Autodesk Inventor part; units mm, degrees
ref_plane "YZ Plane" through (0, 0, 0) normal (1, 0, 0) x (0, 1, 0)
ref_plane "XZ Plane" through (0, 0, 0) normal (0, 1, 0) x (-1, 0, 0)
ref_plane "XY Plane" through (0, 0, 0) normal (0, 0, 1) x (1, 0, 0)
sketch "Sketch3" plane through (0, 0, 0) normal (0, 1, 0) x (-1, 0, 0)
  line L0 (72.5, 90) -> (-72.5, 90)
  line L1 (-72.5, 90) -> (-72.5, -90)
  line L2 (-72.5, -90) -> (72.5, -90)
  line L3 (72.5, -90) -> (72.5, 90)
  line L4 (72.5, 90) -> (-72.5, -90) construction
  line L5 (-72.5, 90) -> (72.5, -90) construction
  point P0 (0, 0)
  dimension "d7" = 145
  dimension "d8" = 180
extrude "Extrusion3" add sketch "Sketch3" along normal blind 5
sketch "Sketch4" plane through (0, 5, 0) normal (0, 1, 0) x (1, 0, 0)
  line L0 (23.935, -64) -> (72.5, -64)
  line L1 (72.5, -64) -> (72.5, -26.408)
  line L2 (72.5, -26.408) -> (23.935, -26.408)
  line L3 (23.935, -26.408) -> (23.935, -64)
  line L4 (23.935, -64) -> (72.5, -26.408) construction
  line L5 (72.5, -64) -> (23.935, -26.408) construction
  line L6 (72.5, -90) -> (72.5, 90)
  line L7 (-72.5, -90) -> (72.5, -90)
  line L8 (-72.5, -64) -> (-23.935, -64)
  line L9 (-23.935, -64) -> (-23.935, -26.408)
  line L10 (-23.935, -26.408) -> (-72.5, -26.408)
  line L11 (-72.5, -26.408) -> (-72.5, -64)
  line L12 (-72.5, -64) -> (-23.935, -26.408) construction
  line L13 (-23.935, -64) -> (-72.5, -26.408) construction
  line L14 (-72.5, 90) -> (-72.5, -90)
  point P0 (0, 0)
  point P1 (48.2175, -45.204)
  point P2 (-48.2175, -45.204)
  dimension "d11" = 48.565
  dimension "d12" = 37.592
  dimension "d13" = 0
  dimension "d14" = 26
  dimension "d20" = 48.565
  dimension "d21" = 37.592
  dimension "d22" = 0
  dimension "d23" = 26
extrude "Extrusion4" cut sketch "Sketch4" against normal blind 2
sketch "Sketch5" plane through (0, 3, 0) normal (0, 1, 0) x (1, 0, 0)
  circle A0 centre (66.797, -60.825) radius 1.588
  line L0 (72.5, -26.408) -> (72.5, -64)
  line L1 (72.5, -64) -> (23.935, -64)
  circle A1 centre (60.447, -60.825) radius 1.588
  circle A2 centre (54.097, -60.825) radius 1.588
  circle A3 centre (47.747, -60.825) radius 1.588
  circle A4 centre (41.397, -60.825) radius 1.588
  circle A5 centre (35.047, -60.825) radius 1.588
  circle A6 centre (28.697, -60.825) radius 1.588
  circle A7 centre (66.797, -29.583) radius 1.588
  circle A8 centre (60.447, -29.583) radius 1.588
  circle A9 centre (54.097, -29.583) radius 1.588
  circle A10 centre (47.747, -29.583) radius 1.588
  circle A11 centre (41.397, -29.583) radius 1.588
  circle A12 centre (35.047, -29.583) radius 1.588
  circle A13 centre (28.697, -29.583) radius 1.588
  circle A14 centre (-66.797, -60.825) radius 1.588
  line L2 (-23.935, -64) -> (-72.5, -64)
  line L3 (-72.5, -64) -> (-72.5, -26.408)
  circle A15 centre (-60.447, -60.825) radius 1.588
  circle A16 centre (-54.097, -60.825) radius 1.588
  circle A17 centre (-47.747, -60.825) radius 1.588
  circle A18 centre (-41.397, -60.825) radius 1.588
  circle A19 centre (-35.047, -60.825) radius 1.588
  circle A20 centre (-28.697, -60.825) radius 1.588
  circle A21 centre (-66.797, -29.583) radius 1.588
  circle A22 centre (-60.447, -29.583) radius 1.588
  circle A23 centre (-54.097, -29.583) radius 1.588
  circle A24 centre (-47.747, -29.583) radius 1.588
  circle A25 centre (-41.397, -29.583) radius 1.588
  circle A26 centre (-35.047, -29.583) radius 1.588
  circle A27 centre (-28.697, -29.583) radius 1.588
  point P0 (0, 0)
  dimension "d24" = 3.176
  dimension "d25" = 5.703
  dimension "d26" = 3.175
  dimension "d30" = 6.35
  dimension "d33" = 31.242
  dimension "d36" = 3.176
  dimension "d37" = 3.175
  dimension "d38" = 5.703
  dimension "d41" = 6.35
  dimension "d44" = 31.242
extrude "Extrusion5" cut sketch "Sketch5" against normal through all
sketch "Sketch6" plane through (0, 5, 0) normal (0, 1, 0) x (1, 0, 0)
  line L0 (42.5, 32.6926) -> (52.5, 32.6926)
  line L1 (52.5, 32.6926) -> (52.5, 37.6926)
  line L2 (52.5, 37.6926) -> (42.5, 37.6926)
  line L3 (42.5, 37.6926) -> (42.5, 32.6926)
  line L4 (42.5, 32.6926) -> (52.5, 37.6926) construction
  line L5 (52.5, 32.6926) -> (42.5, 37.6926) construction
  line L6 (72.5, -26.408) -> (72.5, 90)
  line L7 (-52.5, 32.6926) -> (-42.5, 32.6926)
  line L8 (-42.5, 32.6926) -> (-42.5, 37.6926)
  line L9 (-42.5, 37.6926) -> (-52.5, 37.6926)
  line L10 (-52.5, 37.6926) -> (-52.5, 32.6926)
  line L11 (-52.5, 32.6926) -> (-42.5, 37.6926) construction
  line L12 (-42.5, 32.6926) -> (-52.5, 37.6926) construction
  line L13 (-72.5, 90) -> (-72.5, -26.408)
  line L14 (-52.5, -15.3074) -> (-42.5, -15.3074)
  line L15 (-42.5, -15.3074) -> (-42.5, -12.3074)
  line L16 (-42.5, -12.3074) -> (-52.5, -12.3074)
  line L17 (-52.5, -12.3074) -> (-52.5, -15.3074)
  line L18 (-52.5, -15.3074) -> (-42.5, -12.3074) construction
  line L19 (-42.5, -15.3074) -> (-52.5, -12.3074) construction
  line L20 (42.5, -15.3074) -> (52.5, -15.3074)
  line L21 (52.5, -15.3074) -> (52.5, -12.3074)
  line L22 (52.5, -12.3074) -> (42.5, -12.3074)
  line L23 (42.5, -12.3074) -> (42.5, -15.3074)
  line L24 (42.5, -15.3074) -> (52.5, -12.3074) construction
  line L25 (52.5, -15.3074) -> (42.5, -12.3074) construction
  arc A0 (-42.5, 37.6926) -> (-52.5, 37.6926) centre (-47.5, 37.6926) ccw
  arc A1 (52.5, 37.6926) -> (42.5, 37.6926) centre (47.5, 37.6926) ccw
  line L26 (-72.5, -26.408) -> (-23.935, -26.408)
  line L27 (23.935, -26.408) -> (72.5, -26.408)
  point P0 (0, 0)
  point P1 (47.5, 35.1926)
  point P2 (-47.5, 35.1926)
  point P3 (-47.5, -13.8074)
  point P4 (47.5, -13.8074)
  dimension "d49" = 10
  dimension "d50" = 5
  dimension "d51" = 20
  dimension "d52" = 10
  dimension "d53" = 5
  dimension "d54" = 20
  dimension "d57" = 10
  dimension "d58" = 3
  dimension "d59" = 10
  dimension "d60" = 3
  dimension "d61" = 45
  dimension "d84" = 11.1006
  dimension "d85" = 11.1006
extrude "Extrusion6" add sketch "Sketch6" along normal blind 24
sketch "Sketch7" plane through (0, 5, 0) normal (0, 1, 0) x (1, 0, 0)
  circle A0 centre (62.5, -80) radius 2.5
  line L0 (72.5, -90) -> (72.5, -64)
  line L1 (-72.5, -90) -> (72.5, -90)
  circle A1 centre (-62.5, -80) radius 2.5
  line L2 (-72.5, -64) -> (-72.5, -90)
  circle A2 centre (-39.5, -20.408) radius 2.5
  line L3 (-42.5, -15.3074) -> (-42.5, -12.3074)
  line L4 (-72.5, -26.408) -> (-23.935, -26.408)
  circle A3 centre (39.5, -20.408) radius 2.5
  line L5 (42.5, -12.3074) -> (42.5, -15.3074)
  line L6 (23.935, -26.408) -> (72.5, -26.408)
  line L7 (52.5, 35.6926) -> (42.5, 35.6926)
  circle A4 centre (39.5, -20.408) radius 4
  circle A5 centre (-39.5, -20.408) radius 4
  circle A6 centre (-62.5, -80) radius 4
  circle A7 centre (62.5, -80) radius 4
  circle A8 centre (-10, 77.5) radius 2.5
  line L8 (72.5, 90) -> (-72.5, 90)
  circle A9 centre (10, 77.5) radius 2.5
  point P0 (0, 0)
  point P1 (52.5, 37.6926)
  point P2 (42.5, 37.6926)
  point P3 (0, 90)
  point P4 (0, 90)
  dimension "d63" = 5
  dimension "d64" = 10
  dimension "d65" = 10
  dimension "d66" = 5
  dimension "d67" = 10
  dimension "d68" = 10
  dimension "d69" = 5
  dimension "d70" = 3
  dimension "d71" = 6
  dimension "d72" = 5
  dimension "d73" = 3
  dimension "d74" = 6
  dimension "d80" = 1.5
  dimension "d81" = 1.5
  dimension "d82" = 1.5
  dimension "d83" = 1.5
  dimension "d90" = 5
  dimension "d91" = 12.5
  dimension "d92" = 10
  dimension "d93" = 5
  dimension "d94" = 10
extrude "Extrusion7" cut sketch "Sketch7" against normal through all contours A0 | A1 | A2 | A3 | A8 | A9
sketch "Sketch8" plane through (0, 29, 0) normal (0, 1, 0) x (1, 0, 0)
  line L0 (-42.5, 32.6926) -> (-52.5, 32.6926)
  line L1 (-47.5, 32.6926) -> (-47.5, 42.6926)
  arc A0 (-42.5, 37.6926) -> (-52.5, 37.6926) centre (-47.5, 37.6926) ccw
  line L2 (42.5, 32.6926) -> (52.5, 32.6926)
  line L3 (47.5, 32.6926) -> (47.5, 42.6926)
  arc A1 (52.5, 37.6926) -> (42.5, 37.6926) centre (47.5, 37.6926) ccw
  circle A2 centre (47.5, 37.6926) radius 2.5
  circle A3 centre (-47.5, 37.6926) radius 2.5
  point P0 (0, 0)
  dimension "d86" = 5
  dimension "d87" = 5
extrude "Extrusion8" cut sketch "Sketch8" against normal blind 10
fillet "Fillet1" radius 6 4 edges at (72.5, 2.5, 90) (-72.5, 2.5, 90) (-72.5, 2.5, -90) (72.5, 2.5, -90)
properties part number "chasis"
The listing builds one solid part. Answer for the finished solid, in the listing's coordinates (mm). A direction names the side the tool comes from. Give positions to 0.01 mm unless a question says otherwise; leave off trailing zeros. Order: outer loops, then holes, each group sorted by start corner. A loop starts at its lowest first (then second) coordinate and runs counter-clockwise, first axis right, second up.
1) Determine the mould class of faces 4 (the face through (11.15, 2.54, -75.28)), 5 (the face through (48, 17, 12.307)), 6 (the face through (52.5, 17, -35)), 7 (the face through (-47.61, 16.83, -42.69)) for opening direction X: pulls with the +X half, pulls with the -X half, needs draft (parallel to the pull), parting line crosses it, or undercut.
Reported:
face 4: undercut
face 5: needs draft
face 6: pulls with the +X half
face 7: undercut
2) Find section D-D on z = 75.5. Write down the section's boundary in (x, y), then the cut area to 3 significant figures.
Reported:
outline: (-72.5, 0) - (72.5, 0) - (72.5, 5) - (-72.5, 5) - close
area: 725 mm2
3) Find section C-C on y = 14.25. Write down the section's boundary in (x, z).
Reported:
outline: (-52.5, -37.69) arc R5 ccw to (-42.5, -37.69) - (-42.5, -32.69) - (-52.5, -32.69) - close; (-52.5, 12.31) - (-42.5, 12.31) - (-42.5, 15.31) - (-52.5, 15.31) - close; (42.5, -37.69) arc R5 ccw to (52.5, -37.69) - (52.5, -32.69) - (42.5, -32.69) - close; (42.5, 12.31) - (52.5, 12.31) - (52.5, 15.31) - (42.5, 15.31) - close
4) Find section A-A on z = -77.5. Write down the section's boundary in (x, y).
Reported:
outline: (-72.5, 0) - (-12.5, 0) - (-12.5, 5) - (-72.5, 5) - close; (-7.5, 0) - (7.5, 0) - (7.5, 5) - (-7.5, 5) - close; (12.5, 0) - (72.5, 0) - (72.5, 5) - (12.5, 5) - close
5) Find section B-B on y = 26.25. Write down the section's boundary in (x, z), then the cut area to 3 significant figures.
Reported:
outline: (-52.5, -37.69) arc R5 ccw to (-42.5, -37.69) - (-42.5, -32.69) - (-52.5, -32.69) - close; (-52.5, 12.31) - (-42.5, 12.31) - (-42.5, 15.31) - (-52.5, 15.31) - close; (42.5, -37.69) arc R5 ccw to (52.5, -37.69) - (52.5, -32.69) - (42.5, -32.69) - close; (42.5, 12.31) - (52.5, 12.31) - (52.5, 15.31) - (42.5, 15.31) - close; hole circle Ø5 at (-47.5, -37.69); hole circle Ø5 at (47.5, -37.69)
area: 199 mm2
6) Consider line 1 along Z through (x, y) = (-39.5, 2.25); line 2 along X through (y, z) = (1.85, 80); line 3 along Z through (x, y) = (-47.5, 23.5). Determine where each line is inside the solid, lowest interval first.
Reported:
line 1: z = -90 to 17.91, 22.91 to 90
line 2: x = -72.5 to -65, -60 to 60, 65 to 72.5
line 3: z = -42.69 to -40.19, -35.19 to -32.69, 12.31 to 15.31
7) For faces 1 (the face through (-42.5, 17, -35)), 2 (the face through (47, 17, 15.307)), 3 (the face through (-45.19, 24.07, -36.74)), determine the directions among +Z, -Z, +X, -X, +Y, -Y from which every point of the face is accessible in a straight line to the end or side of a thin tool.
Reported:
face 1: +Z, -Z, +Y
face 2: +Z, +X, -X, +Y
face 3: +Y
8) Given P1, Ø19, axis at x = -48.5, z = 51.5, coming from the +Y side; P2, Ø2.5, axis at x = -66.797, z = 60.825, coming from the -Y side; P3, Ø6, axis at y = 26, z = 11.5, coming from the +X side; P4, Ø12, axis at y = 12, z = 16.5, coming from the -X side, each flat-ended and moving along its own axis, determine where each tip first touches the part or whether it passes through.
Reported:
P1: stops at y = 3
P2: passes through
P3: stops at x = 52.5
P4: stops at x = -52.5
